Design review of the part built by this model. Coordinates are the model's own, in mm. A direction names the side the tool comes from. Coordinates: 2 decimals unless noted, no trailing zeros. Loops run counter-clockwise (first coordinate to the right, second up) from the corner with the lowest first, then second, coordinate; pieces in that order, holes last. Notation, with made-up numbers: M 30,36.25 L 53,36.25 A24 ccw 53,65.25 Z; hole C 44,-2.5 d6. An arc over 180 degrees is marked long. One line per item, written item: value.
```python
from build123d import *

# Parameters (mm, degrees)
SKETCH_W     = 25
SKETCH_H     = 27
PAD_DEPTH    = 2
SKETCH001_W  = 19.3
SKETCH001_H  = 21.2
PAD001_DEPTH = 2
SKETCH002_W  = 1.5
SKETCH002_H  = 20
POCKET_DEPTH = 5
CHAMFER_SIZE = 1.5


with BuildPart() as part:
    # Sketch → Pad (new body)
    with BuildSketch(Plane.XY):
        with Locations((0, 0.1)):
            Rectangle(SKETCH_W, SKETCH_H)
    extrude(amount=PAD_DEPTH)

    # Sketch001 (on Face6 of Pad) → Pad001 (join)
    with BuildSketch(Plane.XY.offset(2)):
        Rectangle(SKETCH001_W, SKETCH001_H)
    extrude(amount=PAD001_DEPTH)

    # Sketch002 (on Face11 of Pad001) → Pocket (cut)
    with BuildSketch(Plane.XY.offset(4)):
        with Locations((1.5, 0)):
            Rectangle(SKETCH002_W, SKETCH002_H)
        with Locations((4.5, 0)):
            Rectangle(SKETCH002_W, SKETCH002_H)
        with Locations((7.5, 0)):
            Rectangle(SKETCH002_W, SKETCH002_H)
        with Locations((-1.5, 0)):
            Rectangle(SKETCH002_W, SKETCH002_H)
        with Locations((-4.5, 0)):
            Rectangle(SKETCH002_W, SKETCH002_H)
        with Locations((-7.5, 0)):
            Rectangle(SKETCH002_W, SKETCH002_H)
    extrude(amount=-POCKET_DEPTH, mode=Mode.SUBTRACT)

    # Chamfer
    chamfer_edges = [part.edges().sort_by_distance(p)[0] for p in [
        (0, 13.6, 0),
        (12.5, 0.1, 0),
        (-12.5, 0.1, 0),
        (0, -13.4, 0),
    ]]
    chamfer(chamfer_edges, length=CHAMFER_SIZE)


solid = part.part
```
(1) We need section A-A on y = 4.5. State how many separate pieces and enclosed holes the cut face has, then the cut area to 4 significant figures.
Reply:
separate pieces: 7
enclosed holes: 0
area: 50.35 mm2
(2) To check wall thickness, follow line 1 along Y through (x, z) = (-1.75, 3.25); line 2 along Y through (x, z) = (-3, 3); line 3 along Y through (x, z) = (9, 1.25). State the ranges of each line that lie inside material, in increasing order. Write a range as [from, to].
Reply:
line 1: y = [-10.6, -10], [10, 10.6]
line 2: y = [-10.6, 10.6]
line 3: y = [-13.15, 13.35]
(3) Insertion check: pin 1 (1.2 mm diameter, centred on y = -0.5, z = 1, fed in from -X); pin 2 (0.8 mm diameter, centred on x = 1, z = 1, fed in from -Y); pin 3 (1 mm diameter, centred on y = 2, z = 3, fed in from -X); pin 4 (1 mm diameter, centred on x = 0.5, z = 3.5, fed in from -Y). Each pin has a flat end and moves straight along its axis. Give the tip position at first contact, or say it passes through.
Reply:
pin 1: stops at x = -12.5
pin 2: stops at y = -13.3
pin 3: stops at x = -9.65
pin 4: stops at y = -10.6
(4) We need section D-D on z = 0.45. State the section outline as (x, y) points, then the cut area to 3 significant figures.
Reply:
outline: M -11.45,-12.35 L 11.45,-12.35 L 11.45,12.55 L -11.45,12.55 Z; hole M -8.25,-10 L -6.75,-10 L -6.75,10 L -8.25,10 Z; hole M -5.25,-10 L -3.75,-10 L -3.75,10 L -5.25,10 Z; hole M -2.25,-10 L -0.75,-10 L -0.75,10 L -2.25,10 Z; hole M 0.75,-10 L 2.25,-10 L 2.25,10 L 0.75,10 Z; hole M 3.75,-10 L 5.25,-10 L 5.25,10 L 3.75,10 Z; hole M 6.75,-10 L 8.25,-10 L 8.25,10 L 6.75,10 Z
area: 390 mm2
(5) Tool access review of faces 1 (the flat face through (0, 10.6, 3)), 2 (the flat face through (0, -10.6, 3)), 3 (the flat face through (-8, 10, 2)): name each direction out of +Z, -Z, +X, -X, +Y, -Y from which nothing blocks a thin tool from reaching the whole face with its end or side.
Reply:
face 1: +Z, +X, -X, +Y
face 2: +Z, +X, -X, -Y
face 3: +Z, -Z
(6) We need section C-C on x = -4.25. State the section outline as (y, z) points.
Reply:
outline: M -13.4,1.5 L -11.9,0 L -10,0 L -10,4 L -10.6,4 L -10.6,2 L -13.4,2 Z; M 10,0 L 12.1,0 L 13.6,1.5 L 13.6,2 L 10.6,2 L 10.6,4 L 10,4 Z
(7) Mouldability with a two-part tool opening along Y and no side actions: class faces 4 (the flat face through (-0.2, 12.8, 0.7)), 5 (the flat face through (-2, -10, 2)), 6 (the flat face through (-9.65, 0, 3)) as released by +Y, released by -Y, zero draft, split by the parting line, or undercut.
Reply:
face 4: released by +Y
face 5: undercut
face 6: zero draft
(8) We need section B-B on z = 2.4. State the section outline as (x, y) points.
Reply:
outline: M -9.65,-10.6 L 9.65,-10.6 L 9.65,10.6 L -9.65,10.6 Z; hole M -8.25,-10 L -6.75,-10 L -6.75,10 L -8.25,10 Z; hole M -5.25,-10 L -3.75,-10 L -3.75,10 L -5.25,10 Z; hole M -2.25,-10 L -0.75,-10 L -0.75,10 L -2.25,10 Z; hole M 0.75,-10 L 2.25,-10 L 2.25,10 L 0.75,10 Z; hole M 3.75,-10 L 5.25,-10 L 5.25,10 L 3.75,10 Z; hole M 6.75,-10 L 8.25,-10 L 8.25,10 L 6.75,10 Z
